Check sheet for the drawn part. Datum: minimum x, y, z corner. Units: mm. A direction names the side the tool comes from. Round coordinates to 2 decimals unless told otherwise and drop trailing zeros. Write each loop counter-clockwise with the first axis right and the second up, starting at its lowest first coordinate (ties: lowest second). Pieces come first, ordered by that corner, then holes. Notation, with made-up numbers: (54.25, -38) -> (63.25, -38) arc R17 ccw to (63.25, -18) -> close; hole circle Ø4 at (84, 68). An arc over 180 degrees is marked (long way). Use a Markdown table: item, result.
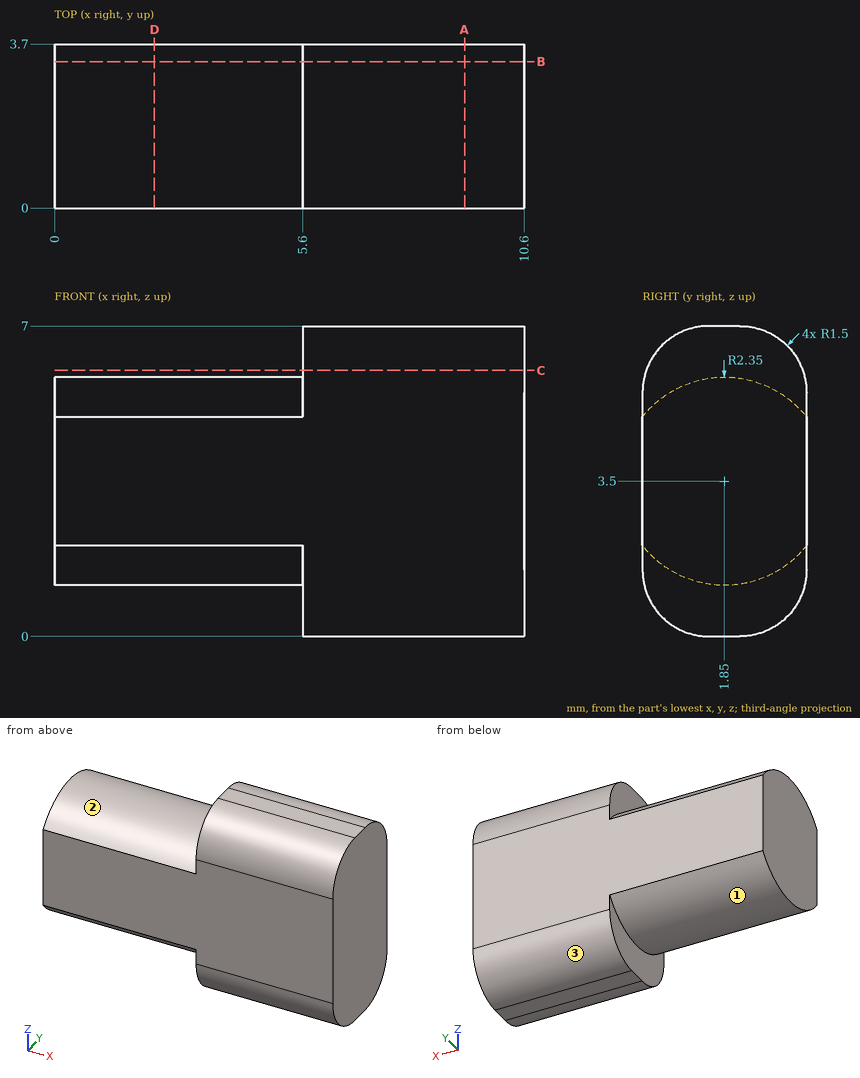
(1) Section check B-B on y = 3.3. Record the cut outline in (x, z), plus the area to 3 significant figures.
A:
| item | result |
|---|---|
| outline | (0, 1.65) -> (5.6, 1.65) -> (5.6, 0.48) -> (10.6, 0.48) -> (10.6, 6.52) -> (5.6, 6.52) -> (5.6, 5.35) -> (0, 5.35) -> close |
| area | 50.9 mm2 |
(2) Thickness scan on line 1 (Z direction, x = 2, y = 1.85); line 2 (X direction, y = 1.9, z = 0.5); line 3 (Y direction, x = 8.5, z = 0.75). Record the ranges inside material, lowest first.
A:
| item | result |
|---|---|
| line 1 | z = 1.15 to 5.85 |
| line 2 | x = 5.6 to 10.6 |
| line 3 | y = 0.2 to 3.5 |
(3) Access from +Z, -Z, +X, -X, +Y, -Y to the whole of each face (thin tool, end or side, straight path). Record for the marked faces 1, 2 and 3.
A:
| item | result |
|---|---|
| face 1 | -Z, -X |
| face 2 | +Z, -X |
| face 3 | -Z, +X, -X, +Y |
(4) Section check C-C on z = 6. Record the cut outline in (x, y), plus the area to 3 significant figures.
A:
| item | result |
|---|---|
| outline | (5.6, 0.09) -> (10.6, 0.09) -> (10.6, 3.61) -> (5.6, 3.61) -> close |
| area | 17.6 mm2 |
(5) Section check D-D on x = 2.25. Record the cut outline in (y, z).
A:
| item | result |
|---|---|
| outline | (0, 2.05) arc R2.35 ccw to (3.7, 2.05) -> (3.7, 4.95) arc R2.35 ccw to (0, 4.95) -> close |
(6) Gauge pin test, flat end, axial feed: pin 1 Ø1.5 at (x, y) = (4, 1) entering from -Z. Record the tip position at first contact, or that the pin passes through.
A:
| item | result |
|---|---|
| pin 1 | stops at z = 1.15 |
(7) Section check A-A on x = 9.25. Record the cut outline in (y, z).
A:
| item | result |
|---|---|
| outline | (0, 1.5) arc R1.5 ccw to (1.5, 0) -> (2.2, 0) arc R1.5 ccw to (3.7, 1.5) -> (3.7, 5.5) arc R1.5 ccw to (2.2, 7) -> (1.5, 7) arc R1.5 ccw to (0, 5.5) -> close |
